Source: CAD feature listing. Evaluate the final solid. Frame: model axes, mm. A direction names the side the tool comes from. Round coordinates to 2 decimals unless told otherwise and drop trailing zeros. Write each loop counter-clockwise with the first axis right and the second up, starting at its lowest first coordinate (ties: lowest second). Pieces come first, ordered by that corner, then holes. Notation, with made-up numbers: M 73.5,9 L 105.5,9 A26 ccw 105.5,38 Z; hole C 29.25,-1 d1. An arc over 180 degrees is marked long. Answer in a Markdown table with one row per item. Add a question column.
Item 1: Contact query for flat-ended pins moving along their axis: pin 1 (7 mm diameter, centred on x = 2, z = 1, fed in from +Y); pin 2 (4.5 mm diameter, centred on x = 0, z = 0, fed in from -Y); pin 3 (1 mm diameter, centred on y = 2, z = 3.5, fed in from +X); pin 4 (3 mm diameter, centred on y = 5, z = -7, fed in from -X). Output: stop coordinate, or through.
Item 2: Cut plane B-B on x = 0. Give the number of separate pieces and of enclosed holes in the cut face, and give its area (3 significant figures).
Item 3: Mould query, pull axis X, two halves, no side actions, for faces 3 (the face through (-1.96, 2.46, -4.63)), 4 (the face through (2, 0, 2)). Classes: released by +X, released by -X, zero draft, split by the parting line, or undercut.
Item 4: Cut plane A-A on y = 5.5. Return loops of the section in (x, z) (3 decimals).
Item 5: Set-up query: faces 1 (the face through (0.78, 2.54, 2.48)), 2 (the face through (0, 5, 3)). Return all of +Z, -Z, +X, -X, +Y, -Y with unobstructed straight access to the full face (end or side cutting, diameter ignored); none if empty.
Item 6: Material intervals for probe 1 along Y at (x, z) = (-4.75, -4.5); probe 2 along X at (y, z) = (2, 4.25); probe 3 along Z at (x, y) = (4, 2.5), sorted ascending.
from build123d import *

# Parameters (mm, degrees)
BOSS_EXTRU_1_DEPTH      = 6.5
ESQUISSE6_R             = 2.6
ENL_V_MAT_EXTRU_2_DEPTH = 15.607361158
ESQUISSE7_R             = 8.5
ENL_V_MAT_EXTRU_4_DEPTH = 1.5
CONG_1_R                = 1.5


with BuildPart() as part:
    # Esquisse1 → Boss.-Extru.1 (new body)
    with BuildSketch(Plane(origin=(0, 0, 0), x_dir=(1, 0, 0), z_dir=(0, 1, 0))):
        with BuildLine():
            ThreePointArc((-4.625, -8.010734985), (0, -9.25), (4.625, -8.010734985))
            ThreePointArc((4.625, -8.010734985), (9.25, 0), (4.625, 8.010734985))
            ThreePointArc((4.625, 8.010734985), (0, 9.25), (-4.625, 8.010734985))
            ThreePointArc((-4.625, 8.010734985), (-9.25, 0), (-4.625, -8.010734985))
        make_face()
    extrude(amount=BOSS_EXTRU_1_DEPTH)

    # Esquisse6 → Enlèv. mat.-Extru.2 (cut, through all)
    with BuildSketch(Plane(origin=(0, 6.5, 0), x_dir=(1, 0, 0), z_dir=(0, 1, 0))):
        with Locations(Location((0, 0, 0), (0, 0, 270))):
            Circle(ESQUISSE6_R)
    extrude(amount=-ENL_V_MAT_EXTRU_2_DEPTH, mode=Mode.SUBTRACT)

    # Esquisse7 → Enlèv. mat.-Extru.4 (cut)
    with BuildSketch(Plane(origin=(0, 6.5, 0), x_dir=(1, 0, 0), z_dir=(0, 1, 0))):
        with Locations(Location((0, 0, 0), (0, 0, 270))):
            Circle(ESQUISSE7_R)
    extrude(amount=-ENL_V_MAT_EXTRU_4_DEPTH, mode=Mode.SUBTRACT)

    # Congé1
    cong_1_edges = [part.edges().sort_by_distance(p)[0] for p in [
        (0, 5, -8.5),
    ]]
    fillet(cong_1_edges, radius=CONG_1_R - 0.0001)  # a hair under: the kernel refuses the full size

    # Enlèv. mat.-Extru.3 cone 1 section (through the dimple's axis) → Enlèv. mat.-Extru.3 (revolve, cut)
    with BuildSketch(Plane(origin=(0, 5, -5.6), x_dir=(0, 0, 1), z_dir=(1, 0, 0))):
        Polygon((0, 0), (0.9, 0), (0, 12.870599631), align=None)
    revolve(axis=Axis((0, 5, -5.6), (0, -1, 0)), mode=Mode.SUBTRACT)

    # Enlèv. mat.-Extru.3 cone 2 section (through the dimple's axis) → Enlèv. mat.-Extru.3 cone 2 (revolve, cut)
    with BuildSketch(Plane(origin=(2.602449763, 5, -4.958553744), x_dir=(0, 0, 1), z_dir=(1, 0, 0))):
        Polygon((0, 0), (0.9, 0), (0, 12.870599631), align=None)
    revolve(axis=Axis((2.602449763, 5, -4.958553744), (0, -1, 0)), mode=Mode.SUBTRACT)

    # Enlèv. mat.-Extru.3 cone 3 section (through the dimple's axis) → Enlèv. mat.-Extru.3 cone 3 (revolve, cut)
    with BuildSketch(Plane(origin=(4.608709649, 5, -3.181162582), x_dir=(0, 0, 1), z_dir=(1, 0, 0))):
        Polygon((0, 0), (0.9, 0), (0, 12.870599631), align=None)
    revolve(axis=Axis((4.608709649, 5, -3.181162582), (0, -1, 0)), mode=Mode.SUBTRACT)

    # Enlèv. mat.-Extru.3 cone 4 section (through the dimple's axis) → Enlèv. mat.-Extru.3 cone 4 (revolve, cut)
    with BuildSketch(Plane(origin=(5.559169695, 5, -0.675005409), x_dir=(0, 0, 1), z_dir=(1, 0, 0))):
        Polygon((0, 0), (0.9, 0), (0, 12.870599631), align=None)
    revolve(axis=Axis((5.559169695, 5, -0.675005409), (0, -1, 0)), mode=Mode.SUBTRACT)

    # Enlèv. mat.-Extru.3 cone 5 section (through the dimple's axis) → Enlèv. mat.-Extru.3 cone 5 (revolve, cut)
    with BuildSketch(Plane(origin=(5.236090959, 5, 1.985787367), x_dir=(0, 0, 1), z_dir=(1, 0, 0))):
        Polygon((0, 0), (0.9, 0), (0, 12.870599631), align=None)
    revolve(axis=Axis((5.236090959, 5, 1.985787367), (0, -1, 0)), mode=Mode.SUBTRACT)

    # Enlèv. mat.-Extru.3 cone 6 section (through the dimple's axis) → Enlèv. mat.-Extru.3 cone 6 (revolve, cut)
    with BuildSketch(Plane(origin=(3.713486886, 5, 4.19166019), x_dir=(0, 0, 1), z_dir=(1, 0, 0))):
        Polygon((0, 0), (0.9, 0), (0, 12.870599631), align=None)
    revolve(axis=Axis((3.713486886, 5, 4.19166019), (0, -1, 0)), mode=Mode.SUBTRACT)

    # Enlèv. mat.-Extru.3 cone 7 section (through the dimple's axis) → Enlèv. mat.-Extru.3 cone 7 (revolve, cut)
    with BuildSketch(Plane(origin=(1.34016772, 5, 5.437274178), x_dir=(0, 0, 1), z_dir=(1, 0, 0))):
        Polygon((0, 0), (0.9, 0), (0, 12.870599631), align=None)
    revolve(axis=Axis((1.34016772, 5, 5.437274178), (0, -1, 0)), mode=Mode.SUBTRACT)

    # Enlèv. mat.-Extru.3 cone 8 section (through the dimple's axis) → Enlèv. mat.-Extru.3 cone 8 (revolve, cut)
    with BuildSketch(Plane(origin=(-1.34016772, 5, 5.437274178), x_dir=(0, 0, 1), z_dir=(1, 0, 0))):
        Polygon((0, 0), (0.9, 0), (0, 12.870599631), align=None)
    revolve(axis=Axis((-1.34016772, 5, 5.437274178), (0, -1, 0)), mode=Mode.SUBTRACT)

    # Enlèv. mat.-Extru.3 cone 9 section (through the dimple's axis) → Enlèv. mat.-Extru.3 cone 9 (revolve, cut)
    with BuildSketch(Plane(origin=(-3.713486886, 5, 4.19166019), x_dir=(0, 0, 1), z_dir=(1, 0, 0))):
        Polygon((0, 0), (0.9, 0), (0, 12.870599631), align=None)
    revolve(axis=Axis((-3.713486886, 5, 4.19166019), (0, -1, 0)), mode=Mode.SUBTRACT)

    # Enlèv. mat.-Extru.3 cone 10 section (through the dimple's axis) → Enlèv. mat.-Extru.3 cone 10 (revolve, cut)
    with BuildSketch(Plane(origin=(-5.236090959, 5, 1.985787367), x_dir=(0, 0, 1), z_dir=(1, 0, 0))):
        Polygon((0, 0), (0.9, 0), (0, 12.870599631), align=None)
    revolve(axis=Axis((-5.236090959, 5, 1.985787367), (0, -1, 0)), mode=Mode.SUBTRACT)

    # Enlèv. mat.-Extru.3 cone 11 section (through the dimple's axis) → Enlèv. mat.-Extru.3 cone 11 (revolve, cut)
    with BuildSketch(Plane(origin=(-5.559169695, 5, -0.675005409), x_dir=(0, 0, 1), z_dir=(1, 0, 0))):
        Polygon((0, 0), (0.9, 0), (0, 12.870599631), align=None)
    revolve(axis=Axis((-5.559169695, 5, -0.675005409), (0, -1, 0)), mode=Mode.SUBTRACT)

    # Enlèv. mat.-Extru.3 cone 12 section (through the dimple's axis) → Enlèv. mat.-Extru.3 cone 12 (revolve, cut)
    with BuildSketch(Plane(origin=(-4.608709649, 5, -3.181162582), x_dir=(0, 0, 1), z_dir=(1, 0, 0))):
        Polygon((0, 0), (0.9, 0), (0, 12.870599631), align=None)
    revolve(axis=Axis((-4.608709649, 5, -3.181162582), (0, -1, 0)), mode=Mode.SUBTRACT)

    # Enlèv. mat.-Extru.3 cone 13 section (through the dimple's axis) → Enlèv. mat.-Extru.3 cone 13 (revolve, cut)
    with BuildSketch(Plane(origin=(-2.602449763, 5, -4.958553744), x_dir=(0, 0, 1), z_dir=(1, 0, 0))):
        Polygon((0, 0), (0.9, 0), (0, 12.870599631), align=None)
    revolve(axis=Axis((-2.602449763, 5, -4.958553744), (0, -1, 0)), mode=Mode.SUBTRACT)


solid = part.part
Results below:
| question | item | result |
|---|---|---|
| 1 | pin 1 | y = 5 |
| 1 | pin 2 | through |
| 1 | pin 3 | x = 8.75 |
| 1 | pin 4 | x = -7.44 |
| 2 | separate pieces | 3 |
| 2 | enclosed holes | 0 |
| 2 | area | 62.5 mm2 |
| 3 | face 3 | undercut |
| 3 | face 4 | zero draft |
| 4 | outline | C 0,0 d18.5; hole C 0,0 d16.236 |
| 5 | face 1 | +Y, -Y |
| 5 | face 2 | +Y |
| 6 | probe 1 | 0 to 5 |
| 6 | probe 2 | -8.22 to -4.4, -3.03 to 3.03, 4.4 to 8.22 |
| 6 | probe 3 | -8.34 to -3.58, -2.79 to 3.53, 4.86 to 8.34 |
